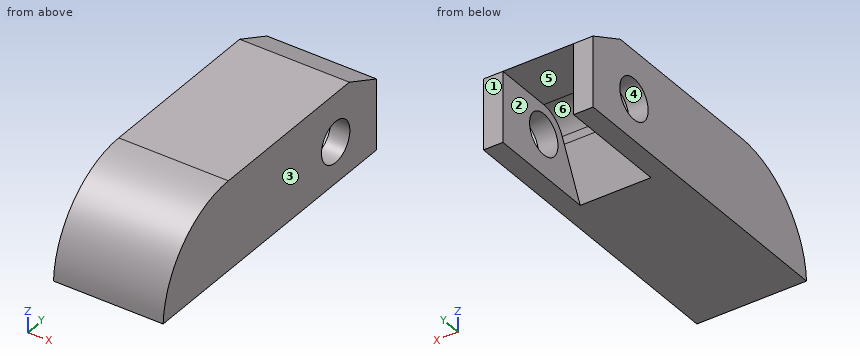
from build123d import *

# Parameters (mm, degrees)
SKETCH1_W               = 11.811
SKETCH1_H               = 45.98924
BOSS_EXTRUDE1_DEPTH     = 9.652
FILLET5_R               = 4.826
SKETCH2_W               = 7.62
SKETCH2_H               = 22.352
CUT_EXTRUDE1_DEPTH      = 7.62
CUT_EXTRUDE2_DEPTH      = 49.452771033
CUT_EXTRUDE2_DEPTH_BACK = 49.452771033
SKETCH3_R               = 2.20345
FILLET4_R               = 4.826
FILLET6_R               = 10.16
CUT_EXTRUDE3_DEPTH      = 49.452771033
CUT_EXTRUDE4_DEPTH      = 7.62
BOSS_EXTRUDE2_DEPTH     = 7.62


with BuildPart() as part:
    # Sketch1 → Boss-Extrude1 (new body)
    with BuildSketch(Plane.XY):
        with Locations((5.9055, 22.99462)):
            Rectangle(SKETCH1_W, SKETCH1_H)
    extrude(amount=BOSS_EXTRUDE1_DEPTH)

    # Fillet5
    fillet5_edges = [part.edges().sort_by_distance(p)[0] for p in [
        (5.9055, 45.98924, 0),
    ]]
    fillet(fillet5_edges, radius=FILLET5_R)

    # Sketch2 → Cut-Extrude1 (cut)
    with BuildSketch(Plane(origin=(0, 0, 0), x_dir=(-1, 0, 0), z_dir=(0, 0, -1))):
        with Locations((-5.9055, 34.81324)):
            Rectangle(SKETCH2_W, SKETCH2_H)
    extrude(amount=-CUT_EXTRUDE1_DEPTH, mode=Mode.SUBTRACT)

    # Sketch3 → Cut-Extrude2 (cut, two sides: drawn at the far end of the back side and taken through both)
    with BuildSketch(Plane.ZY.offset(-CUT_EXTRUDE2_DEPTH_BACK)):
        with Locations((4.4323, 26.82494)):
            Circle(SKETCH3_R)
    extrude(amount=CUT_EXTRUDE2_DEPTH + CUT_EXTRUDE2_DEPTH_BACK, mode=Mode.SUBTRACT)

    # Fillet4
    # the kernel refuses this fillet: 4.826 mm, written as the material it takes off along each edge
    with BuildSketch(Plane(origin=(23.876, 45.98924, 9.652), x_dir=(0, 0, -1), z_dir=(-1, 0, 0))) as fillet4_piece_1:
        with BuildLine():
            CenterArc((FILLET4_R, FILLET4_R), FILLET4_R, 180, 90)
            Line((0, FILLET4_R), (0, 0))
            Line((0, 0), (FILLET4_R, 0))
        make_face()
    extrude(amount=35.941, mode=Mode.SUBTRACT)

    # Fillet6
    # the kernel refuses this fillet: 10.16 mm, written as the material it takes off along each edge
    with BuildSketch(Plane(origin=(-25.368230131, 0, 9.652), x_dir=(0, 1, 0), z_dir=(1, 0, 0))) as fillet6_piece_1:
        with BuildLine():
            CenterArc((10.147292053, -10.16), FILLET6_R, 90, 87.134016017)
            Line((0, -9.652), (-0.202945841, -9.64184))
            ThreePointArc((-0.202945841, -9.64184), (-0.2032, -4.826), (-0.2032, 0))
            Line((-0.2032, 0), (0, 0.2032))
            Line((0, 0.2032), (10.147292053, 0.2032))
            Line((10.147292053, 0.2032), (10.147292053, 0))
        make_face()
    extrude(amount=62.547460263, mode=Mode.SUBTRACT)

    # Sketch4 → Cut-Extrude3 (cut, through all)
    with BuildSketch(Plane(origin=(11.811, 0, 0), x_dir=(0, 0, -1), z_dir=(1, 0, 0))):
        Polygon((-9.652, 28.943813088), (-7.62, 33.17494), (0, 33.17494), (0, 45.98924), (-9.652, 45.98924), align=None)
    extrude(amount=-CUT_EXTRUDE3_DEPTH, mode=Mode.SUBTRACT)

    # Sketch5 → Cut-Extrude4 (cut)
    with BuildSketch(Plane.ZY.offset(-9.7155)):
        Polygon((0, 21.160076085), (5.158068358, 23.63724), (0, 23.63724), align=None)
    extrude(amount=CUT_EXTRUDE4_DEPTH, mode=Mode.SUBTRACT)

    # Sketch5<3> → Boss-Extrude2 (add)
    with BuildSketch(Plane.ZY.offset(-9.7155)):
        with BuildLine():
            Line((5.812301369, 23.951435604), (5.158068358, 23.63724))
            Line((5.158068358, 23.63724), (7.62, 23.63724))
            Line((7.62, 23.63724), (7.62, 26.82494))
            ThreePointArc((7.62, 26.82494), (7.130490287, 25.127530072), (5.812301369, 23.951435604))
        make_face()
    extrude(amount=BOSS_EXTRUDE2_DEPTH)


solid = part.part
Build history of the part. All positions in model axes, mm. Face numbers are marked on the shaded views. A direction names the side the tool comes from. Round coordinates to 2 decimals unless told otherwise and drop trailing zeros. Write each loop counter-clockwise with the first axis right and the second up, starting at its lowest first coordinate (ties: lowest second). Pieces come first, ordered by that corner, then holes. Notation, with made-up numbers: (2, 7) - (42, 7) arc R9 cw to (42, 19) - close; hole circle Ø4 at (89.25, 15). An arc over 180 degrees is marked (long way). Use CSV: the item, a comma, the result in double quotes.
(1) Band-saw the part on C-C (z = 0.75). Write the cut outline in (x, y).
Response:
outline,"(0, 0.07) - (11.81, 0.07) - (11.81, 33.17) - (9.72, 33.17) - (9.72, 21.52) - (2.1, 21.52) - (2.1, 33.17) - (0, 33.17) - close"
(2) Band-saw the part on B-B (z = 3.25). Write the cut outline in (x, y).
Response:
outline,"(0, 0.71) - (11.81, 0.71) - (11.81, 24.97) - (9.72, 24.97) - (9.72, 22.72) - (2.1, 22.72) - (2.1, 24.97) - (0, 24.97) - close; (0, 28.68) - (2.1, 28.68) - (2.1, 33.17) - (0, 33.17) - close; (9.72, 28.68) - (11.81, 28.68) - (11.81, 33.17) - (9.72, 33.17) - close"
(3) Band-saw the part on A-A (x = 7). Write the cut outline in (y, z).
Response:
outline,"(0, 0) - (21.16, 0) - (23.95, 5.81) arc R3.19 cw to (26.82, 7.62) - (33.17, 7.62) - (28.94, 9.65) - (10.15, 9.65) arc R10.16 ccw to start"
(4) 3-axis set-ups, long thin cutter, end or side, ignore diameter. For the marked faces 1 and 2: which of +Z, -Z, +X, -X, +Y, -Y reach the whole face in a straight line?
Response:
face 1,"+Z, -Z, +X, -X, +Y"
face 2,"-Z, +Y"
(5) Band-saw the part on D-D (y = 3.5). Write the cut outline in (x, z).
Response:
outline,"(0, 0) - (11.81, 0) - (11.81, 7.18) - (0, 7.18) - close"
(6) Pin check, flat tip, straight feed: P1, Ø5, axis at y = 26.82, z = 4.43, coming from the +X side. Stop position of the tip, or through.
Response:
P1,"x = 11.81"
(7) Mould opens along X. For the marked faces 3, 4, 5 and 6 say: pulls with the +X half, pulls with the -X half, needs draft (parallel to the pull), parting line crosses it, or undercut.
Response:
face 3,"pulls with the +X half"
face 4,"needs draft"
face 5,"undercut"
face 6,"undercut"
(8) Wall check: line 1 (X direction, y = 30, z = 2.5); line 2 (Z direction, x = 8.75, y = 7); line 3 (Y direction, x = 5.5, z = 4.5). Give the ranges that are in metal, low to high.
Response:
line 1,"0 to 2.1, 9.72 to 11.81"
line 2,"0 to 9.15"
line 3,"1.31 to 23.32"
